Here's the drawing with two shaded views (mm, measured from the low corner). I have some questions. A direction names the side the tool comes from. Round coordinates to 2 decimals unless told otherwise and drop trailing zeros. Loops run counter-clockwise (first coordinate to the right, second up) from the corner with the lowest first, then second, coordinate; pieces in that order, holes last.
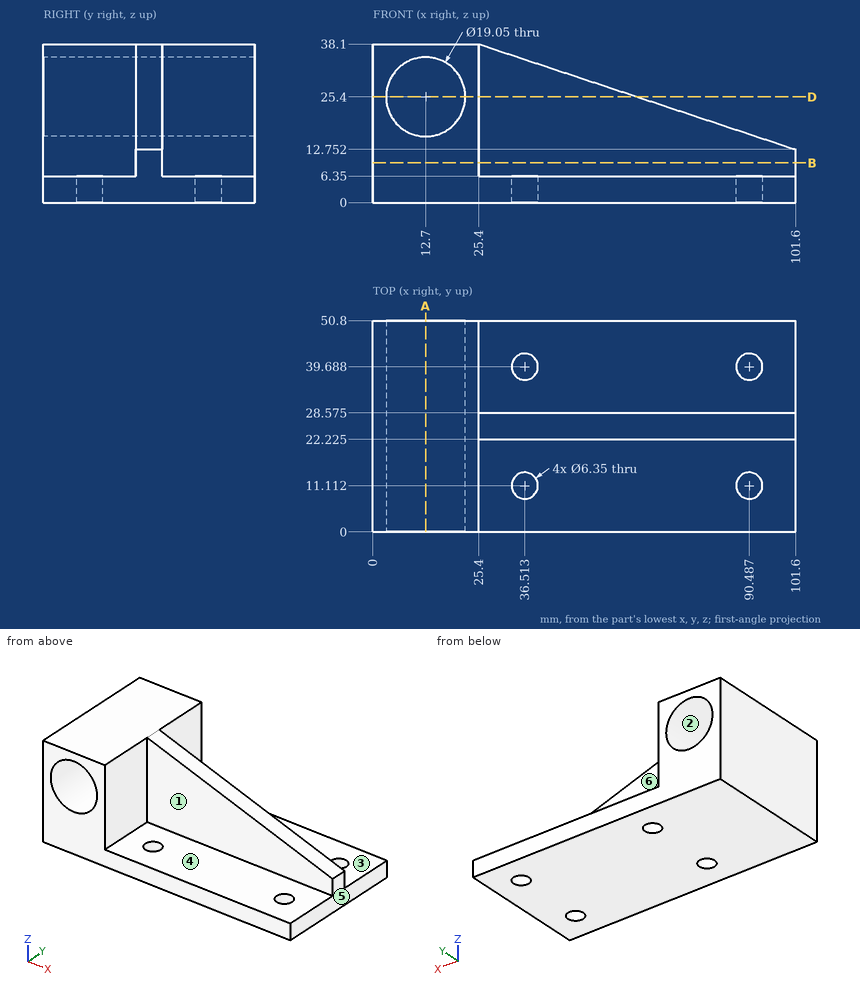
Item 1: We'd pull the mould along Z, two halves only. Please class the marked faces 1, 2 and 3: released by +Z, released by -Z, zero draft, split by the parting line, or undercut.
Results list:
face 1: zero draft
face 2: undercut
face 3: released by +Z
Item 2: If I drill on line 1 along Z through (x, y) = (12.7, 35.5) (1 decimal); line 2 along Z through (x, y) = (46, 42); line 3 along Y through (x, z) = (41, 32) (1 decimal), over which ranges is the centre line in solid material (lowest first)?
Results list:
line 1: z = 0 to 15.9, 34.9 to 38.1
line 2: z = 0 to 6.35
line 3: y = 22.2 to 28.6
Item 3: Will these pins go through, and if not, where does the flat tip stop? pin 1 (18 mm diameter, centred on x = 44.5, y = 13, fed in from +Z); pin 2 (8 mm diameter, centred on x = 29.5, z = 29.5, fed in from -Y) (1 decimal); pin 3 (6.5 mm diameter, centred on y = 13.5, z = 17.5, fed in from +X).
Results list:
pin 1: stops at z = 6.35
pin 2: stops at y = 22.2
pin 3: stops at x = 25.4
Item 4: If we section it at B-B, the plane z = 9.5: Please give me the cut outline in (x, y) (1 decimal), then the cut area to 3 significant figures.
Results list:
outline: (0, 0) - (25.4, 0) - (25.4, 22.2) - (101.6, 22.2) - (101.6, 28.6) - (25.4, 28.6) - (25.4, 50.8) - (0, 50.8) - close
area: 1,770 mm2
Item 5: If we section it at A-A, the plane x = 12.7: Please give me the cut outline in (y, z) (1 decimal).
Results list:
outline: (0, 0) - (50.8, 0) - (50.8, 15.9) - (0, 15.9) - close; (0, 34.9) - (50.8, 34.9) - (50.8, 38.1) - (0, 38.1) - close
Item 6: For the marked faces 4, 5 and 6, which set-ups out of +Z, -Z, +X, -X, +Y, -Y let a thin tool reach every point of the face, with its end or its side?
Results list:
face 4: +Z, +X, -Y
face 5: +Z, -Z, +X, +Y, -Y
face 6: +Z, +X, +Y
Item 7: If we section it at D-D, the plane z = 25.4: Please give me the cut outline in (x, y) (1 decimal), then the cut area to 3 significant figures.
Results list:
outline: (0, 0) - (3.2, 0) - (3.2, 50.8) - (0, 50.8) - close; (22.2, 0) - (25.4, 0) - (25.4, 22.2) - (63.6, 22.2) - (63.6, 28.6) - (25.4, 28.6) - (25.4, 50.8) - (22.2, 50.8) - close
area: 565 mm2
